Verification items for the finished model (mm, model axes). Face numbers are marked on the shaded views. A direction names the side the tool comes from. Coordinates: 2 decimals unless noted, no trailing zeros. Loops run counter-clockwise (first coordinate to the right, second up) from the corner with the lowest first, then second, coordinate; pieces in that order, holes last. Notation, with made-up numbers: (-11, -36) -> (38, -36) arc R15 cw to (38, -12) -> close; hole circle Ø2 at (53.5, 87). An arc over 180 degrees is marked (long way). Answer as a JSON object with one key per item and string values. Group by question number.
Q1. Scan lines: L1, parallel to Y at x = 2, z = -15.5; L2, parallel to Z at x = 18.5, y = -6.5 (3 decimals); L3, parallel to X at y = -9.25, z = -12.5. Record each from-to range of solid material in increasing order.
Q2. Cross-section at A-A on z = 3. Record the boundary of the cut face in (x, y), and give its area (3 significant figures).
Q3. Set-up check for the marked faces 1 and 2: record each of +Z, -Z, +X, -X, +Y, -Y from which the full face is reachable in a straight line by a thin tool's end or side.
Q4. Cross-section at B-B on x = 4.5. Record the boundary of the cut face in (y, z) (3 decimals), and give its area (3 significant figures).
Q5. Cross-section at C-C on x = 17.75. Record the boundary of the cut face in (y, z) (3 decimals), and give its area (3 significant figures).
Q6. Release check for a two-part mould opening along Z. For the marked faces 3, 4 and 5 record: released by +Z, released by -Z, zero draft, split by the parting line, or undercut.
Q7. Gauge pin test, flat ends, axial feed: pin 1 Ø1 at (y, z) = (-2, -17) entering from -X; pin 2 Ø4 at (x, y) = (7, 8.5) entering from -Z (3 decimals); pin 3 Ø12 at (x, y) = (4.5, 0.5) entering from -Z (3 decimals). Record the tip position at first contact, or that the pin passes through.
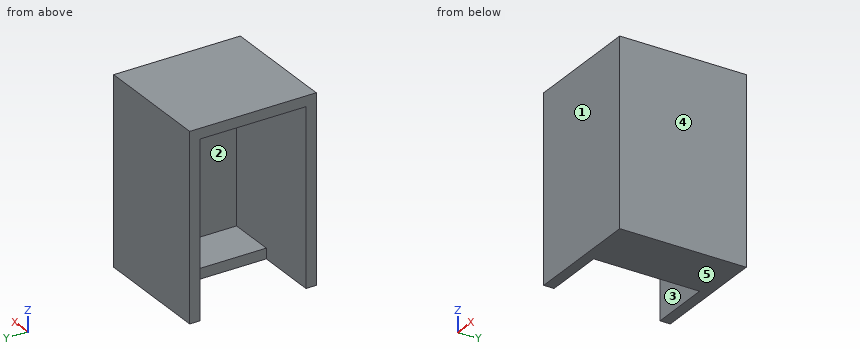
```python
from build123d import *

# Parameters (mm, degrees)
SKETCH4_W           = 31.75
SKETCH4_H           = 20.5
BOSS_EXTRUDE1_DEPTH = 21
SHELL1_T            = 2
SKETCH5_W           = 12
SKETCH5_H           = 20.5
CUT_EXTRUDE1_DEPTH  = 2


with BuildPart() as part:
    # Sketch4 → Boss-Extrude1 (new body)
    with BuildSketch(Plane(origin=(0, 0, 0), x_dir=(0, 0, -1), z_dir=(1, 0, 0))):
        Rectangle(SKETCH4_W, SKETCH4_H)
    extrude(amount=BOSS_EXTRUDE1_DEPTH)

    # Shell1
    shell1_openings = [part.faces().sort_by_distance(p)[0] for p in [
        (0, 0, 0),
    ]]
    offset(amount=SHELL1_T, openings=shell1_openings, kind=Kind.INTERSECTION)

    # Sketch5 → Cut-Extrude1 (cut)
    with BuildSketch(Plane(origin=(0, 0, -17.875), x_dir=(-1, 0, 0), z_dir=(0, 0, -1))):
        with Locations((-6, 0)):
            Rectangle(SKETCH5_W, SKETCH5_H)
    extrude(amount=-CUT_EXTRUDE1_DEPTH, mode=Mode.SUBTRACT)


solid = part.part
```
Computed values:
{
 "1": {"L1": "y = -12.25 to -10.25, 10.25 to 12.25", "L2": "z = -17.875 to -15.875, 15.875 to 17.875", "L3": "x = 21 to 23"},
 "2": {"outline": "(0, -12.25) -> (23, -12.25) -> (23, 12.25) -> (0, 12.25) -> (0, 10.25) -> (21, 10.25) -> (21, -10.25) -> (0, -10.25) -> close", "area": "133 mm²"},
 "3": {"face 1": "+Z, -Z, +X, -X, -Y", "face 2": "-X"},
 "4": {"outline": "(-12.25, -17.875) -> (-10.25, -17.875) -> (-10.25, 15.875) -> (10.25, 15.875) -> (10.25, -17.875) -> (12.25, -17.875) -> (12.25, 17.875) -> (-12.25, 17.875) -> close", "area": "184 mm²"},
 "5": {"outline": "(-12.25, -17.875) -> (12.25, -17.875) -> (12.25, 17.875) -> (-12.25, 17.875) -> close; hole (-10.25, -15.875) -> (10.25, -15.875) -> (10.25, 15.875) -> (-10.25, 15.875) -> close", "area": "225 mm²"},
 "6": {"face 3": "undercut", "face 4": "zero draft", "face 5": "released by -Z"},
 "7": {"pin 1": "stops at x = 12", "pin 2": "stops at z = -17.875", "pin 3": "stops at z = 15.875"}
}
